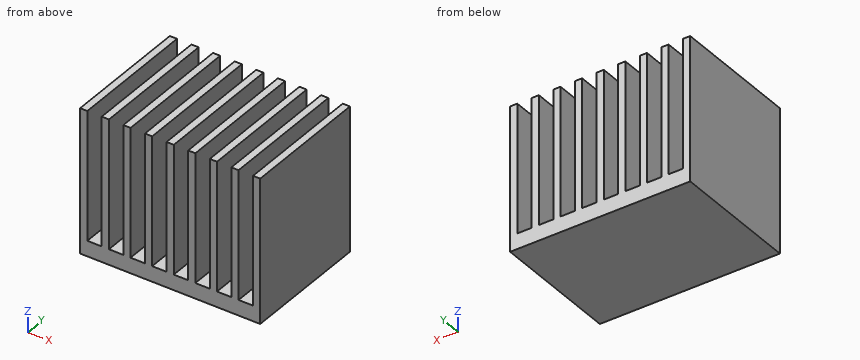
from build123d import *

# Parameters (mm, degrees)
F0_W     = 8.89
F0_H     = 6.35
F1_DEPTH = 0.762
F2_W     = 0.3556
F2_H     = 6.35
F3_DEPTH = 6.35


with BuildPart() as f1:
    # F0 (on Top) → F1 (new body)
    with BuildSketch(Plane.XY):
        Rectangle(F0_W, F0_H)
    extrude(amount=F1_DEPTH)

    # F2 (on face) → F3 (join)
    with BuildSketch(Plane.XY.offset(0.762)):
        with Locations((-4.2672, 0)):
            Rectangle(F2_W, F2_H)
        with Locations((-3.2004, 0)):
            Rectangle(F2_W, F2_H)
        with Locations((-2.1336, 0)):
            Rectangle(F2_W, F2_H)
        with Locations((-1.0668, 0)):
            Rectangle(F2_W, F2_H)
        Rectangle(F2_W, F2_H)
        with Locations((1.0668, 0)):
            Rectangle(F2_W, F2_H)
        with Locations((2.1336, 0)):
            Rectangle(F2_W, F2_H)
        with Locations((3.2004, 0)):
            Rectangle(F2_W, F2_H)
        with Locations((4.2672, 0)):
            Rectangle(F2_W, F2_H)
    extrude(amount=F3_DEPTH)


solid = f1.part
For this review, take the finished solid that the model builds, in its own axes (mm). Round coordinates to 2 decimals unless told otherwise and drop trailing zeros. Order: outer loops, then holes, each group sorted by start corner. A loop starts at its lowest first (then second) coordinate and runs counter-clockwise, first axis right, second up. Notation, with made-up numbers: (78, 81.25) -> (93, 81.25) arc R25 cw to (93, 116.25) -> close; hole circle Ø8 at (-25.5, -6.5). An arc over 180 degrees is marked (long way). Put each result on its own line as item: value.
Q1. Add section A-A on z = 2.25. State how many separate pieces and enclosed holes the cut face has, plus the area to 3 significant figures.
Check result:
separate pieces: 9
enclosed holes: 0
area: 20.3 mm2
Q2. Add section B-B on x = -0.75. Write out the cut boundary in (y, z) (3 decimals), plus the area to 3 significant figures.
Check result:
outline: (-3.175, 0) -> (3.175, 0) -> (3.175, 0.762) -> (-3.175, 0.762) -> close
area: 4.84 mm2
Q3. For probe 1 along Z at (x, y) = (2.5, 2), list the stretches that pass through material, from the lowest coordinate up. Write a range as [from, to].
Check result:
probe 1: [0, 0.76]
